Design review of the part shown in the three views and the two pictorial views. Dimensions are in mm from the part's minimum x, y and z. Coordinates: 2 decimals unless noted, no trailing zeros. Order: outer loops, then holes, each group sorted by start corner. A loop starts at its lowest first (then second) coordinate and runs counter-clockwise, first axis right, second up. Notation, with made-up numbers: (89.5, 28) -> (99.5, 28) arc R20 cw to (99.5, 50) -> close; hole circle Ø3 at (21.25, 50). An arc over 180 degrees is marked (long way). Answer as CSV lines item,"result". Start each with the question number.
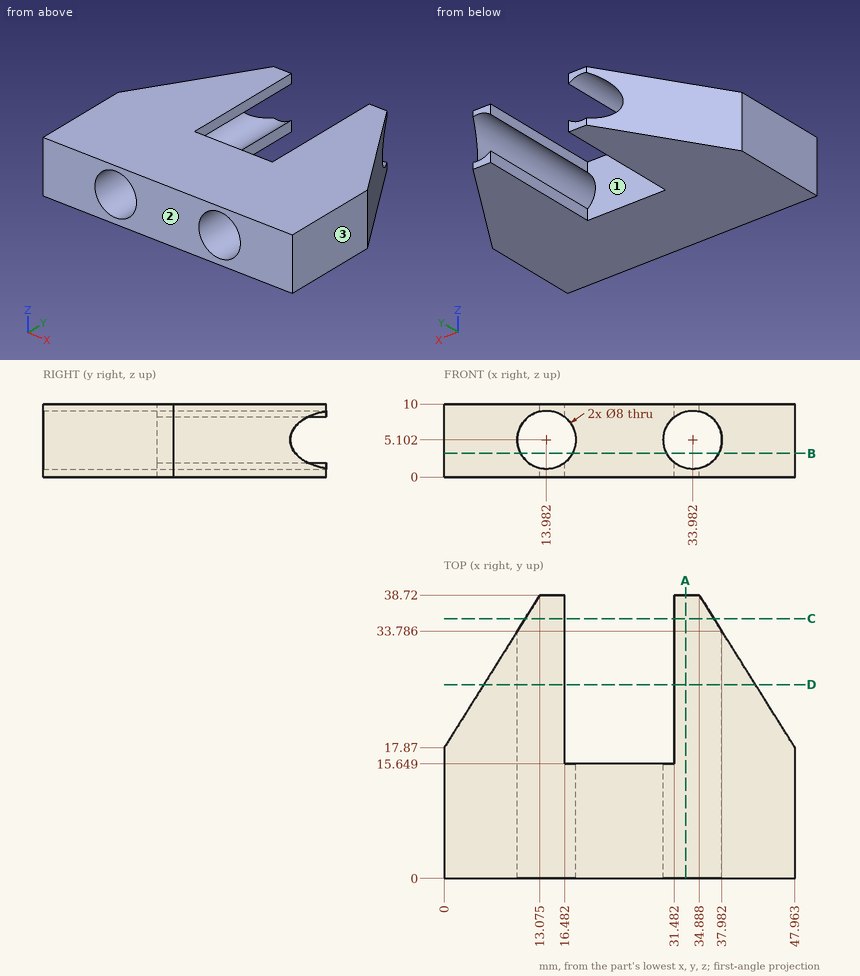
1) Insertion check: pin 1 Ø0.5 at (y, z) = (23, 9.5) entering from +X; pin 2 Ø3 at (x, z) = (24.5, 5.5) entering from +Y; pin 3 Ø0.9 at (y, z) = (32, 9.5) entering from -X. Each pin has a flat end and moves straight along its axis. Give the tip position at first contact, or say it passes through.
2) Wall thickness on L1, parallel to X at y = 8, z = 6.75 (1 decimal); L2, parallel to X at y = 6.5, z = 5.5; L3, parallel to Z at x = 32, y = 25 (1 decimal): over which ranges is each line inside the solid? List them lowest first. Write a range as [from, to].
3) Consider section C-C (y = 35.5). Give the boundary of the cut face in (x, z) (1 decimal).
4) Consider section B-B (z = 3.25). Give the boundary of the cut face in (x, y).
5) Consider section A-A (x = 33). Give the boundary of the cut face in (y, z) (1 decimal).
6) Mouldability with a two-part tool opening along X and no side actions: class the marked faces 1, 2 and 3 as released by +X, released by -X, zero draft, split by the parting line, or undercut.
7) Consider section D-D (y = 26.5). Give the boundary of the cut face in (x, z) (1 decimal), plus the area to 3 significant figures.
Result:
1,pin 1,"x = 44.9"
1,pin 2,"y = 15.65"
1,pin 3,"x = 8.58"
2,L1,"[0, 10.3], [17.6, 30.3], [37.6, 48]"
2,L2,"[0, 10], [17.96, 30], [37.96, 47.96]"
2,L3,"[0, 1.6], [8.6, 10]"
3,outline,"(11.1, 0) -> (16.5, 0) -> (16.5, 2) arc R4 cw to (11.1, 2.4) -> close; (11.1, 7.8) arc R4 cw to (16.5, 8.2) -> (16.5, 10) -> (11.1, 10) -> close; (31.5, 0) -> (36.9, 0) -> (36.9, 2.4) arc R4 cw to (31.5, 2) -> close; (31.5, 8.2) arc R4 cw to (36.9, 7.8) -> (36.9, 10) -> (31.5, 10) -> close"
4,outline,"(0, 0) -> (10.44, 0) -> (10.44, 34.51) -> (0, 17.87) -> close; (17.53, 0) -> (30.44, 0) -> (30.44, 15.65) -> (17.53, 15.65) -> close; (37.53, 0) -> (47.96, 0) -> (47.96, 17.87) -> (37.53, 34.51) -> close"
5,outline,"(0, 0) -> (38.7, 0) -> (38.7, 1.2) -> (0, 1.2) -> close; (0, 9) -> (38.7, 9) -> (38.7, 10) -> (0, 10) -> close"
6,face 1,"undercut"
6,face 2,"zero draft"
6,face 3,"released by +X"
7,outline,"(5.4, 0) -> (16.5, 0) -> (16.5, 2) arc R4 cw (long way) to (16.5, 8.2) -> (16.5, 10) -> (5.4, 10) -> close; (31.5, 0) -> (42.6, 0) -> (42.6, 10) -> (31.5, 10) -> (31.5, 8.2) arc R4 cw (long way) to (31.5, 2) -> close"
7,area,"134 mm2"
